from build123d import *

# Parameters (mm, degrees)
F0_R     = 1.5
F1_DEPTH = 3


with BuildPart() as f1:
    # F0 (on Front) → F1 (new body)
    with BuildSketch(Plane.XZ):
        with BuildLine():
            Line((0, -5), (42.227316, -5))
            Line((42.227316, -5), (90, -5))
            ThreePointArc((90, -5), (95, 0), (90, 5))
            Line((90, 5), (45, 5))
            Line((45, 5), (21.213203, 5))
            Line((21.213203, 5), (3.535534, 22.67767))
            Line((3.535534, 22.67767), (-7.071068, 12.071068))
            Line((-7.071068, 12.071068), (-5, 10))
            Line((-5, 10), (-5, 0))
            ThreePointArc((-5, 0), (-3.535534, -3.535534), (0, -5))
        make_face()
        Circle(F0_R, mode=Mode.SUBTRACT)
        with Locations((7.227316, 0)):
            Circle(F0_R, mode=Mode.SUBTRACT)
        with Locations((17.227316, 0)):
            Circle(F0_R, mode=Mode.SUBTRACT)
        with Locations((27.227316, 0)):
            Circle(F0_R, mode=Mode.SUBTRACT)
        with Locations((37.227316, 0)):
            Circle(F0_R, mode=Mode.SUBTRACT)
        with Locations((90, 0)):
            Circle(F0_R, mode=Mode.SUBTRACT)
    extrude(amount=F1_DEPTH)


solid = f1.part
Geometry: final body of the model. Coordinates: model frame, mm. A direction names the side the tool comes from. Give positions to 0.01 mm unless a question says otherwise; leave off trailing zeros. Write each loop counter-clockwise with the first axis right and the second up, starting at its lowest first coordinate (ties: lowest second). Pieces come first, ordered by that corner, then holes. Notation, with made-up numbers: M 10,-16.75 L 34,-16.75 A28 ccw 34,11.25 Z; hole C 48,-39 d7. An arc over 180 degrees is marked long. Answer in a Markdown table with one row per item. Add a question column.
(1) Mould query, pull axis X, two halves, no side actions, for faces 4 (the cylindrical face through (8.6, -1.5, -0.6)), 5 (the cylindrical face through (95, -1, 0)), 6 (the cylindrical face through (-4, -1, -3)). Classes: +X half, -X half, draft (parallel to the pull), parting line (faces both ways), or undercut.
(2) First-contact query: pin 1 (1.5 mm diameter, centred on y = -2, z = 6.5, fed in from -X); pin 2 (2.5 mm diameter, centred on x = 90, z = 0, fed in from -Y) (3 decimals); pin 3 (1 mm diameter, centred on y = -2, z = 6.5, fed in from +X); pin 4 (1.5 mm diameter, centred on x = 44, y = -1, fed in from +Z). Flat tips, straight axial feed; report the tip coordinate or a pass-through.
(3) Section C-C on z = 17.25. Return loops of the section in (x, y).
(4) Section A-A on y = -0.5. Return loops of the section in (x, z), and give its area (3 significant figures).
(5) Ray query, line 1 (Z direction, x = 90, y = -1.3); line 2 (Z direction, x = 82.5, y = -1.3); line 3 (Z direction, x = 8, y = -2.8). Return the intervals inside material, ascending.
(6) Section B-B on x = 59.5. Return loops of the section in (y, z), and give its area (3 significant figures).
(7) Reachability of faces 1 (the cylindrical face through (35.73, -1.48, 0.07)), 2 (the flat face through (56, -1, 5)), 3 (the flat face through (-5, -1, 5)) from +Z, -Z, +X, -X, +Y, -Y: full face, straight path, thin tool, end or side. Return the list, or none.
Result set:
| question | item | result |
|---|---|---|
| 1 | face 4 | undercut |
| 1 | face 5 | +X half |
| 1 | face 6 | -X half |
| 2 | pin 1 | stops at x = -5 |
| 2 | pin 2 | passes through |
| 2 | pin 3 | stops at x = 20.21 |
| 2 | pin 4 | stops at z = 5 |
| 3 | outline | M -1.89,-3 L 8.96,-3 L 8.96,0 L -1.89,0 Z |
| 4 | outline | M -7.07,12.07 L -5,10 L -5,0 A5 ccw 0,-5 L 90,-5 A5 ccw 90,5 L 21.21,5 L 3.54,22.68 Z; hole C 0,0 d3; hole C 7.23,0 d3; hole C 17.23,0 d3; hole C 27.23,0 d3; hole C 37.23,0 d3; hole C 90,0 d3 |
| 4 | area | 1,220 mm^2 |
| 5 | line 1 | z = -5 to -1.5, 1.5 to 5 |
| 5 | line 2 | z = -5 to 5 |
| 5 | line 3 | z = -5 to -1.29, 1.29 to 18.21 |
| 6 | outline | M -3,-5 L 0,-5 L 0,5 L -3,5 Z |
| 6 | area | 30.0 mm^2 |
| 7 | face 1 | +Y, -Y |
| 7 | face 2 | +Z, +X, +Y, -Y |
| 7 | face 3 | -Z, -X, +Y, -Y |
